Autodesk Inventor part; units mm, degrees
ref_plane "YZ Plane" through (0, 0, 0) normal (1, 0, 0) x (0, 1, 0)
ref_plane "XZ Plane" through (0, 0, 0) normal (0, 1, 0) x (-1, 0, 0)
ref_plane "XY Plane" through (0, 0, 0) normal (0, 0, 1) x (1, 0, 0)
sketch "Sketch2" plane through (0, 0, 0) normal (0, 1, 0) x (-1, 0, 0)
  line L0 (0, 0) -> (250, 0)
  line L1 (250, 0) -> (250, -300)
  line L2 (250, -300) -> (0, -300)
  line L3 (0, -300) -> (0, 0)
  dimension "d4" = 250
  dimension "d5" = 300
extrude "Extrusion2" add sketch "Sketch2" along normal blind 5
fillet "Fillet1" radius 2 4 edges at (0, 2.5, 0) (-250, 2.5, 0) (-250, 2.5, -300) (0, 2.5, -300)
sketch "Sketch5" plane through (0, 5, 0) normal (0, 1, 0) x (1, 0, 0)
  line L0 (-2, 300) -> (-248, 300)
  circle A0 centre (-10, 10) radius 5
  circle A1 centre (-10, 290) radius 5
  circle A2 centre (-240, 290) radius 5
  circle A3 centre (-240, 10) radius 5
  point P0 (0, 0)
  point P1 (-15, 150)
  dimension "d25" = 150
hole "Hole1" at (-240, 5, -10) at (-10, 5, -10) at (-10, 5, -290) at (-240, 5, -290) direction (0, -1, 0) diameter 8 depth 25 tip angle 118
sketch "Sketch6" plane through (0, 5, 0) normal (0, 1, 0) x (1, 0, 0)
  circle A0 centre (-142.8286, 250) radius 15
  line L0 (-2, 300) -> (-248, 300)
  circle A1 centre (-142.8286, 250) radius 20
  line L1 (-133.6124, 232.25) -> (-133.6124, 196.3478)
  line L2 (-152.0448, 232.25) -> (-152.0448, 196.3478)
  line L3 (-214.8824, 196.3478) -> (-74.8824, 196.3478)
  line L4 (-74.8824, 196.3478) -> (-74.8824, 291.3478)
  line L5 (-74.8824, 291.3478) -> (-214.8824, 291.3478)
  line L6 (-214.8824, 291.3478) -> (-214.8824, 196.3478)
  point P0 (0, 0)
  dimension "d33" = 30
  dimension "d34" = 50
  dimension "d35" = 40
  dimension "d36" = 140
  dimension "d37" = 95
extrude "Extrusion5" cut sketch "Sketch6" against normal blind 50 contours A0 | A1 L2 L3 L6 L5 L4 L1
sketch "Sketch8" plane through (0, 5, 0) normal (0, 1, 0) x (1, 0, 0)
  line L0 (-152.0448, 196.3478) -> (-214.8824, 196.3478)
  line L1 (-133.6124, 196.3478) -> (-74.8824, 196.3478)
  point P0 (0, 0)
  point P1 (-174.2431, 196.3478)
  point P2 (-174.3182, 73.8636)
  point P3 (-109.2711, 196.3478)
  point P4 (-109.3182, 73.8636)
  dimension "d47" = 65
hole "Hole3" at (-174.3182, 5, -73.8636) at (-109.3182, 5, -73.8636) direction (0, -1, 0) diameter 6 depth 25 tip angle 118
properties part number "bevel desk (hole)" material "Lead"
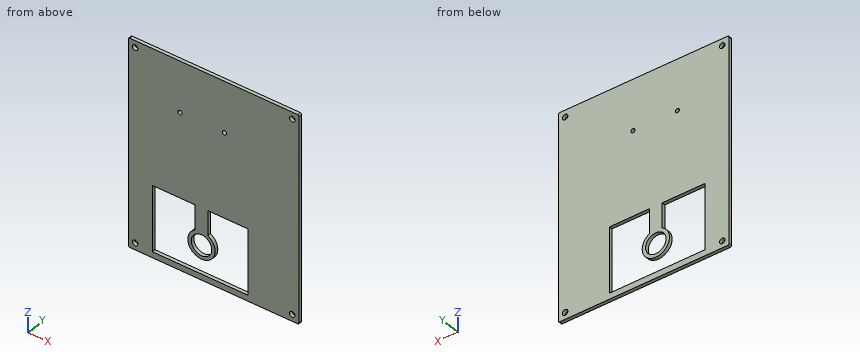
Part model, mm, in its own coordinate system. Give positions to 0.01 mm unless a question says otherwise; leave off trailing zeros. Loops run counter-clockwise (first coordinate to the right, second up) from the corner with the lowest first, then second, coordinate; pieces in that order, holes last. Notation, with made-up numbers: M 44.25,21 L 93.25,21 A28 ccw 93.25,43 Z; hole C -4,-35.5 d5. An arc over 180 degrees is marked long. Put each result on its own line as item: value. Start each with the question number.
1) Saw through at A-A (z = -10). List the corners of the cut face in (x, y), then the cut area to 3 significant figures.
2) Saw through at B-B (x = -10). List the corners of the cut face in (y, z).
3) Saw through at D-D (z = -250). List the corners of the cut face in (x, y), then the cut area to 3 significant figures.
4) Saw through at C-C (x = -190). List the corners of the cut face in (y, z).
5) Probe probe 1 along X at (y, z) = (1.55, -250); probe 2 along X at (y, z) = (1.2, -10); probe 3 along X at (y, z) = (3.2, -274). List the from-to ranges inside material, lowest first.
Numbers:
1. outline: M -250,0 L -244,0 L -244,5 L -250,5 Z; M -236,0 L -14,0 L -14,5 L -236,5 Z; M -6,0 L 0,0 L 0,5 L -6,5 Z
1. area: 1,170 mm^2
2. outline: M 0,-300 L 5,-300 L 5,-294 L 0,-294 Z; M 0,-286 L 5,-286 L 5,-14 L 0,-14 Z; M 0,-6 L 5,-6 L 5,0 L 0,0 Z
3. outline: M -250,0 L -214.88,0 L -214.88,5 L -250,5 Z; M -162.83,0 L -157.83,0 L -157.83,5 L -162.83,5 Z; M -127.83,0 L -122.83,0 L -122.83,5 L -127.83,5 Z; M -74.88,0 L 0,0 L 0,5 L -74.88,5 Z
3. area: 600 mm^2
4. outline: M 0,-300 L 5,-300 L 5,-291.35 L 0,-291.35 Z; M 0,-196.35 L 5,-196.35 L 5,0 L 0,0 Z
5. probe 1: -250 to -214.88, -162.83 to -157.83, -127.83 to -122.83, -74.88 to 0
5. probe 2: -250 to -244, -236 to -14, -6 to 0
5. probe 3: -250 to -214.88, -74.88 to 0
